Build history of the part. All positions in model axes, mm. A direction names the side the tool comes from. Give positions to 0.01 mm unless a question says otherwise; leave off trailing zeros. Order: outer loops, then holes, each group sorted by start corner. A loop starts at its lowest first (then second) coordinate and runs counter-clockwise, first axis right, second up. Notation, with made-up numbers: (65, -31) -> (108, -31) arc R22 cw to (108, 0) -> close; hole circle Ø4 at (76, 53). An arc over 180 degrees is marked (long way). One line per item, written item: value. Start each with the question number.
(1) Saw through at C-C on z = 18. Give the cut face in (x, y), plus the area to 3 significant figures.
(2) Saw through at D-D on y = 22. Give the cut face in (x, z).
(3) Pin check, flat tips, straight feed: pin 1 (10.5 mm diameter, centred on x = 29.5, z = 13, fed in from +Y); pin 2 (1 mm diameter, centred on y = 7.5, z = 3.5, fed in from -X); pin 3 (4 mm diameter, centred on y = 18, z = 14, fed in from +X); pin 4 (6 mm diameter, centred on x = -0.5, y = 14.5, fed in from -Z). Stop position of each tip, or through.
(4) Which spindle directions (+Z, -Z, +X, -X, +Y, -Y) get a long thin tool onto all of the face, cutting with end or side? Do faces 1 (the flat face through (-35, -21, 10)), 2 (the flat face through (20, 5, 10)), 3 (the flat face through (-20, 5, 10)). Say none if no direction does.
(5) Two-plate mould, pull along Y, no slides. Class faces 4 (the flat face through (0, -11, 20)), 5 (the flat face through (0, 25.5, 10)), 6 (the flat face through (0, -25.5, 10)), 7 (the cylindrical face through (-1.953, 20.372, 9.86)): +Y half, -Y half, draft (parallel to the pull), parting line (faces both ways), or undercut.
(6) Probe line 1 (Y direction, x = 0, z = 15.75); line 2 (X direction, y = 14, z = 14); line 3 (X direction, y = 18.5, z = 9.5). List the from-to ranges inside material, lowest first.
(7) Saw through at B-B on y = 5.5. Give the cut face in (x, z), plus the area to 3 significant figures.
(8) Saw through at A-A on x = 0. Give the cut face in (y, z).
```python
from build123d import *

# Parameters (mm, degrees)
F0_R     = 15
F0_W     = 15
F0_H     = 10
F1_DEPTH = 20
F2_F1_R  = 1
F2_F2_R  = 1
F3_R     = 1


with BuildPart() as f1:
    # F0 (on Top) → F1 (new body)
    with BuildSketch(Plane.XY):
        Polygon((-20, -25.5), (20, -25.5), (20, -15.5), (20, 25.5), (-20, 25.5), (-20, -15.5), align=None)
        with Locations((0, 5.5)):
            Circle(F0_R, mode=Mode.SUBTRACT)
        with Locations((-27.5, -20.5)):
            Rectangle(F0_W, F0_H)
        with Locations((27.5, -20.5)):
            Rectangle(F0_W, F0_H)
    extrude(amount=F1_DEPTH)

    # F2: fillet of radius 1 on 10 edges, made by hand

    # F2_f1
    f2_f1_edges = [f1.edges().sort_by_distance(p)[0] for p in [
        (-20, -15.5, 10),
        (20, -15.5, 10),
    ]]
    fillet(f2_f1_edges, radius=F2_F1_R)

    # F2_f2
    f2_f2_edges = [f1.edges().sort_by_distance(p)[0] for p in [
        (-20, 25.5, 10),
        (-20, 5.5, 0),
        (-20, 5.5, 20),
        (20, 25.5, 10),
        (0, 25.5, 0),
        (0, 25.5, 20),
        (20, 5.5, 0),
        (20, 5.5, 20),
        (20.2928932188, -15.2071067812, 20),
        (20.2928932188, -15.2071067812, 0),
        (-20.2928932188, -15.2071067812, 20),
        (-20.2928932188, -15.2071067812, 0),
    ]]
    fillet(f2_f2_edges, radius=F2_F2_R)

    # F3
    f3_edges = [f1.edges().sort_by_distance(p)[0] for p in [
        (21, -15.5, 10),
        (28, -15.5, 1),
        (28, -15.5, 19),
        (35, -15.5, 10),
        (35, -15.792893, 0.292893),
        (35, -15.792893, 19.707107),
        (35, -21, 0),
        (35, -21, 20),
        (35, -25.5, 10),
        (-21, -15.5, 10),
        (-28, -15.5, 1),
        (-28, -15.5, 19),
        (-35, -15.5, 10),
        (-35, -15.792893, 0.292893),
        (-35, -15.792893, 19.707107),
        (-35, -21, 0),
        (-35, -21, 20),
        (-35, -25.5, 10),
    ]]
    fillet(f3_edges, radius=F3_R)


solid = f1.part
```
Results below:
1. outline: (-35, -24.5) arc R1 ccw to (-34, -25.5) -> (34, -25.5) arc R1 ccw to (35, -24.5) -> (35, -16.5) arc R1 ccw to (34, -15.5) -> (21, -15.5) arc R1 cw to (20, -14.5) -> (20, 24.5) arc R1 ccw to (19, 25.5) -> (-19, 25.5) arc R1 ccw to (-20, 24.5) -> (-20, -14.5) arc R1 cw to (-21, -15.5) -> (-34, -15.5) arc R1 ccw to (-35, -16.5) -> close; hole circle Ø30 at (0, 5.5)
1. area: 1,630 mm²
2. outline: (-20, 1) arc R1 ccw to (-19, 0) -> (19, 0) arc R1 ccw to (20, 1) -> (20, 19) arc R1 ccw to (19, 20) -> (-19, 20) arc R1 ccw to (-20, 19) -> close
3. pin 1: stops at y = -15.5
3. pin 2: stops at x = -20
3. pin 3: stops at x = 20
3. pin 4: passes through
4. face 1: +Z, -Z, -X, +Y, -Y
4. face 2: +Z, -Z, +X, +Y
4. face 3: +Z, -Z, -X, +Y
5. face 4: draft
5. face 5: +Y half
5. face 6: -Y half
5. face 7: undercut
6. line 1: y = -25.5 to -9.5, 20.5 to 25.5
6. line 2: x = -20 to -12.36, 12.36 to 20
6. line 3: x = -20 to -7.48, 7.48 to 20
7. outline: (-20, 1) arc R1 ccw to (-19, 0) -> (-15, 0) -> (-15, 20) -> (-19, 20) arc R1 ccw to (-20, 19) -> close; (15, 0) -> (19, 0) arc R1 ccw to (20, 1) -> (20, 19) arc R1 ccw to (19, 20) -> (15, 20) -> close
7. area: 199 mm²
8. outline: (-25.5, 0) -> (-9.5, 0) -> (-9.5, 20) -> (-25.5, 20) -> close; (20.5, 0) -> (24.5, 0) arc R1 ccw to (25.5, 1) -> (25.5, 19) arc R1 ccw to (24.5, 20) -> (20.5, 20) -> close
